```python
from build123d import *

# Parameters (mm, degrees)
SKETCH1_W            = 600
SKETCH1_H            = 1310
SKETCH1_W_2          = 549.2
SKETCH1_H_2          = 1259.2
BOSS_EXTRUDE1_DEPTH  = 2
SKETCH2_W            = 340
SKETCH2_H            = 1310
SKETCH2_W_2          = 289.2
SKETCH2_H_2          = 1259.2
BOSS_EXTRUDE2_DEPTH  = 2
SKETCH3_W            = 340
SKETCH3_H            = 600
SKETCH3_W_2          = 289.2
SKETCH3_H_2          = 549.2
BOSS_EXTRUDE3_DEPTH  = 2
SKETCH4_W            = 2
SKETCH4_H            = 1310
BOSS_EXTRUDE4_DEPTH  = 30
SKETCH5_W            = 2
SKETCH5_H            = 600
BOSS_EXTRUDE8_DEPTH  = 30
SKETCH8_W            = 2
SKETCH8_H            = 30
BOSS_EXTRUDE9_DEPTH  = 30
BOSS_EXTRUDE10_DEPTH = 2
SKETCH10_W           = 15.4
SKETCH10_H           = 60
CUT_EXTRUDE2_DEPTH   = 55
SKETCH11_R           = 4
CUT_EXTRUDE3_DEPTH   = 10


with BuildPart() as part:
    # Sketch1 → Boss-Extrude1 (new body)
    with BuildSketch(Plane(origin=(0, 0, 0), x_dir=(0, 0, -1), z_dir=(1, 0, 0))):
        Rectangle(SKETCH1_W, SKETCH1_H)
        Rectangle(SKETCH1_W_2, SKETCH1_H_2, mode=Mode.SUBTRACT)
    extrude(amount=BOSS_EXTRUDE1_DEPTH)

    # Sketch2 → Boss-Extrude2 (add)
    with BuildSketch(Plane.XY.offset(300)):
        with Locations((-168, 0)):
            Rectangle(SKETCH2_W, SKETCH2_H)
        with Locations((-168, 0)):
            Rectangle(SKETCH2_W_2, SKETCH2_H_2, mode=Mode.SUBTRACT)
    boss_extrude2 = extrude(amount=-BOSS_EXTRUDE2_DEPTH)

    # Sketch3 → Boss-Extrude3 (add)
    with BuildSketch(Plane(origin=(0, 655, 0), x_dir=(1, 0, 0), z_dir=(0, 1, 0))):
        with Locations((-168, 0)):
            Rectangle(SKETCH3_W, SKETCH3_H)
        with Locations((-168, 0)):
            Rectangle(SKETCH3_W_2, SKETCH3_H_2, mode=Mode.SUBTRACT)
    boss_extrude3 = extrude(amount=-BOSS_EXTRUDE3_DEPTH)

    # Mirror3: Boss-Extrude3 across plane
    add(boss_extrude3.mirror(Plane.ZX))

    # Mirror4: Boss-Extrude2 across plane
    add(boss_extrude2.mirror(Plane.XY))


with BuildPart() as body_2:
    # Sketch4 → Boss-Extrude4 (new body)
    with BuildSketch(Plane.XY.offset(300)):
        with Locations((-337, 0)):
            Rectangle(SKETCH4_W, SKETCH4_H)
    extrude(amount=BOSS_EXTRUDE4_DEPTH)


with BuildPart() as body_3:
    # Sketch5 → Boss-Extrude8 (new body)
    with BuildSketch(Plane(origin=(0, 655, 0), x_dir=(1, 0, 0), z_dir=(0, 1, 0))):
        with Locations((-337, 0)):
            Rectangle(SKETCH5_W, SKETCH5_H)
    extrude(amount=BOSS_EXTRUDE8_DEPTH)


with BuildPart() as body_4:
    # Sketch8 → Boss-Extrude9 (new body)
    with BuildSketch(Plane(origin=(0, 655, 0), x_dir=(1, 0, 0), z_dir=(0, 1, 0))):
        with Locations((-337, -315)):
            Rectangle(SKETCH8_W, SKETCH8_H)
    extrude(amount=BOSS_EXTRUDE9_DEPTH)


with BuildPart() as body_5:
    # Sketch9 → Boss-Extrude10 (new body)
    with BuildSketch(Plane.XY.offset(300)):
        Polygon((-336, 685), (-306, 655), (-336, 655), align=None)
    extrude(amount=-BOSS_EXTRUDE10_DEPTH)


with BuildPart() as body_6:
    # Mirror2: mirrored copy
    add(body_3.part.mirror(Plane.ZX))


with BuildPart() as body_7:
    # Mirror2 2: mirrored copy
    add(body_5.part.mirror(Plane.ZX))


with BuildPart() as body_8:
    # Mirror2 3: mirrored copy
    add(body_4.part.mirror(Plane.ZX))


with BuildPart() as body_9:
    # Mirror5: mirrored copy
    add(body_5.part.mirror(Plane.XY))


with BuildPart() as body_10:
    # Mirror5 2: mirrored copy
    add(body_4.part.mirror(Plane.XY))


with BuildPart() as body_11:
    # Mirror5 3: mirrored copy
    add(body_2.part.mirror(Plane.XY))


with BuildPart() as body_12:
    # Mirror5 4: mirrored copy
    add(body_7.part.mirror(Plane.XY))


with BuildPart() as body_13:
    # Mirror5 5: mirrored copy
    add(body_8.part.mirror(Plane.XY))


with BuildPart() as cut_extrude2_tool:
    # Sketch10 → Cut-Extrude2 (new body)
    with BuildSketch(Plane(origin=(0, 685, 0), x_dir=(1, 0, 0), z_dir=(0, 1, 0))):
        with Locations((-330.3, 220)):
            Rectangle(SKETCH10_W, SKETCH10_H)
    extrude(amount=-CUT_EXTRUDE2_DEPTH)


with BuildPart() as part_1:
    add(part.part)

    # Cut-Extrude2: cut by cut_extrude2_tool
    add(cut_extrude2_tool.part, mode=Mode.SUBTRACT)


with BuildPart() as body_3_1:
    add(body_3.part)

    # Cut-Extrude2: cut by cut_extrude2_tool
    add(cut_extrude2_tool.part, mode=Mode.SUBTRACT)


with BuildPart() as cut_extrude3_tool:
    # Sketch11 → Cut-Extrude3 (new body)
    with BuildSketch(Plane(origin=(-336, 0, 0), x_dir=(0, 0, -1), z_dir=(1, 0, 0))):
        with Locations(Location((315, 635, 0), (0, 0, 90))):
            Circle(SKETCH11_R)
        with Locations(Location((315, 0, 0), (0, 0, 90))):
            Circle(SKETCH11_R)
        with Locations(Location((315, -635, 0), (0, 0, 90))):
            Circle(SKETCH11_R)
        with Locations(Location((-315, -635, 0), (0, 0, 90))):
            Circle(SKETCH11_R)
        with Locations(Location((-315, 0, 0), (0, 0, 90))):
            Circle(SKETCH11_R)
        with Locations(Location((-315, 635, 0), (0, 0, 90))):
            Circle(SKETCH11_R)
    extrude(amount=-CUT_EXTRUDE3_DEPTH)


with BuildPart() as body_2_1:
    add(body_2.part)

    # Cut-Extrude3: cut by cut_extrude3_tool
    add(cut_extrude3_tool.part, mode=Mode.SUBTRACT)


with BuildPart() as body_11_1:
    add(body_11.part)

    # Cut-Extrude3: cut by cut_extrude3_tool
    add(cut_extrude3_tool.part, mode=Mode.SUBTRACT)


with BuildPart() as part_2:
    add(part_1.part)

    # Combine1: read off the stored shape, not the designer's step
    # Combine1: union body 3, body 12, body 10, body 13, body 6, body 8, body 4, body 2, body 11, body 9, body 7, body 5
    add(body_3_1.part)
    add(body_12.part)
    add(body_10.part)
    add(body_13.part)
    add(body_6.part)
    add(body_8.part)
    add(body_4.part)
    add(body_2_1.part)
    add(body_11_1.part)
    add(body_9.part)
    add(body_7.part)
    add(body_5.part)


solid = part_2.part
```
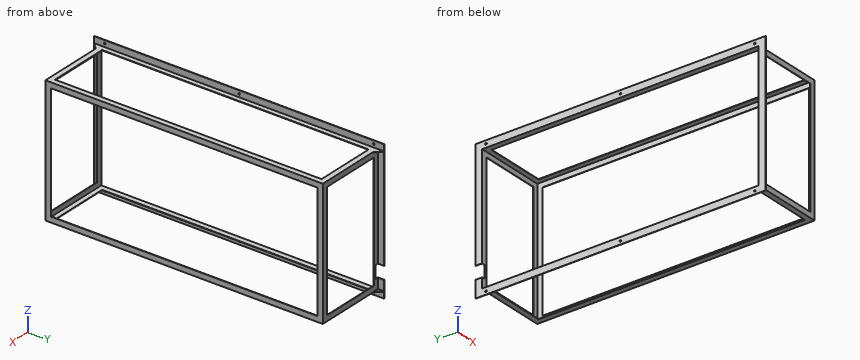
Verification items for the finished model (mm, model axes). Give positions to 0.01 mm unless a question says otherwise; leave off trailing zeros. Loops run counter-clockwise (first coordinate to the right, second up) from the corner with the lowest first, then second, coordinate; pieces in that order, holes last.
1. Section check A-A, the plane z = -175.5. Enter the section's corners in (x, y), then the cut area to 3 significant figures.
2. Go/stop test with flat-tipped pins: pin 1 Ø1.6 at (x, y) = (-159.5, 653.5) entering from -Z; pin 2 Ø7 at (y, z) = (-635, -315) entering from +X; pin 3 Ø9 at (y, z) = (676, 92.5) entering from +X. Record where each tip stops, or that it passes through.
3. Section check B-B, the plane y = -383. Enter the section's corners in (x, z).
4. Thickness scan on line 1 (Y direction, x = -337.4, z = 315); line 2 (Z direction, x = -336.9, y = -635); line 3 (Y direction, x = -138.5, z = 293.5). Record the ranges inside material, lowest first.
Geometry says:
1. outline: (-338, -685) - (-336, -685) - (-336, -655) - (-312.6, -655) - (-312.6, -653) - (-338, -653) - close; (-338, 653) - (-312.6, 653) - (-312.6, 655) - (-336, 655) - (-336, 685) - (-338, 685) - close; (-23.4, -655) - (2, -655) - (2, -629.6) - (0, -629.6) - (0, -653) - (-23.4, -653) - close; (-23.4, 653) - (0, 653) - (0, 629.6) - (2, 629.6) - (2, 655) - (-23.4, 655) - close
1. area: 417 mm2
2. pin 1: stops at z = -300
2. pin 2: passes through
2. pin 3: stops at x = -336
3. outline: (-338, -330) - (-336, -330) - (-336, -300) - (-312.6, -300) - (-312.6, -298) - (-338, -298) - close; (-338, 298) - (-312.6, 298) - (-312.6, 300) - (-336, 300) - (-336, 330) - (-338, 330) - close; (-23.4, -300) - (2, -300) - (2, -274.6) - (0, -274.6) - (0, -298) - (-23.4, -298) - close; (-23.4, 298) - (0, 298) - (0, 274.6) - (2, 274.6) - (2, 300) - (-23.4, 300) - close
4. line 1: y = -685 to -639, -631 to -4, 4 to 631, 639 to 685
4. line 2: z = -330 to -319, -311 to -298, 298 to 311, 319 to 330
4. line 3: y = -655 to -653, 653 to 655
